Can you work these out from the model? Positions are in its coordinate system, mm. Give positions to 0.01 mm unless a question says otherwise; leave off trailing zeros. Write each loop counter-clockwise with the first axis right and the second up, starting at its lowest first coordinate (ties: lowest second). Pieces come first, ordered by that corner, then holes.
Solid Edge part; units mm, degrees
sketch "Sketch1" plane through (0, 0, 0) normal (0, -1, 0) x (1, 0, 0)
  circle A0 centre (-39.1274, 31.1489) radius 2.5
  line L0 (40.6726, 22.6489) -> (-39.1274, 22.6489)
  line L1 (-39.1274, 39.6489) -> (40.6726, 39.6489)
  arc A1 (-39.1274, 22.6489) -> (-39.1274, 39.6489) centre (-39.1274, 31.1489) cw
  arc A2 (40.6726, 39.6489) -> (40.6726, 22.6489) centre (40.6726, 31.1489) cw
  circle A3 centre (40.6726, 31.1489) radius 2.5
extrude "Protrusion1" add sketch "Sketch1" against normal blind 1
1) Suppose I cut it at C-C on z = 37.5. Write out the boundary of the cut face in (x, y), plus the area to 3 significant figures.
Values follow:
outline: (-44.78, 0) - (46.32, 0) - (46.32, 1) - (-44.78, 1) - close
area: 91.1 mm2
2) Suppose I cut it at B-B on y = 0.65. Write out the boundary of the cut face in (x, z), plus the area to 3 significant figures.
Values follow:
outline: (-39.13, 22.65) - (40.67, 22.65) arc R8.5 ccw to (40.67, 39.65) - (-39.13, 39.65) arc R8.5 ccw to start; hole circle Ø5 at (-39.13, 31.15); hole circle Ø5 at (40.67, 31.15)
area: 1,540 mm2
3) For pin 1 Ø6.5 at (x, z) = (-39.13, 31.15) entering from +Y, with a flat end and sliding along its axis, tell me the tip position at first contact or that it passes through.
Values follow:
pin 1: stops at y = 1
4) If we mould it in two halves opening along X, with no side actions, what happens to faces 1 (the face through (1, 0, 31)), 2 (the face through (49.17, 0.49, 30.96)), 3 (the face through (38.83, 0.49, 32.84))? For each: +X half, -X half, draft (parallel to the pull), parting line (faces both ways), or undercut.
Values follow:
face 1: draft
face 2: +X half
face 3: undercut
5) Suppose I cut it at D-D on z = 26. Write out the boundary of the cut face in (x, y).
Values follow:
outline: (-45.89, 0) - (47.44, 0) - (47.44, 1) - (-45.89, 1) - close
6) Suppose I cut it at A-A on z = 30. Write out the boundary of the cut face in (x, y).
Values follow:
outline: (-47.55, 0) - (-41.35, 0) - (-41.35, 1) - (-47.55, 1) - close; (-36.91, 0) - (38.45, 0) - (38.45, 1) - (-36.91, 1) - close; (42.89, 0) - (49.09, 0) - (49.09, 1) - (42.89, 1) - close
7) Please list where these lines run through material, in increasing order: L1, parallel to X at y = 0.5, z = 33; L2, parallel to X at y = 0.15, z = 29.5; L3, parallel to X at y = 0.85, z = 24.25.
Values follow:
L1: x = -47.42 to -40.81, -37.45 to 38.99, 42.35 to 48.97
L2: x = -47.47 to -41.01, -37.25 to 38.79, 42.55 to 49.01
L3: x = -44.09 to 45.64
